The figure shows three views and two pictorial views of one solid part (mm, origin at its lowest corner). Answer the questions. A direction names the side the tool comes from. Coordinates: 2 decimals unless noted, no trailing zeros. Write each loop counter-clockwise with the first axis right and the second up, starting at its lowest first coordinate (ties: lowest second). Pieces come first, ordered by that corner, then holes.
Item 1: Section C-C (x = 63.5) is taken. Give the vertices of the cut face in (y, z), then the cut area to 3 significant figures.
Item 2: Section B-B (z = 24) is taken. Give the vertices of the cut face in (x, y), then the cut area to 3 significant figures.
Item 3: Each of these flat-tipped pins is pushed along its axis until it touches: P1, Ø16.5, axis at x = 12.7, y = 12.7, coming from the +Z side; P2, Ø2, axis at x = 53, z = 43.5, coming from the +Y side; P3, Ø10, axis at y = 47.5, z = 36.5, coming from the +X side. Where does it stop, or does it pass through?
Item 4: Determine the mould class of the marked faces 1, 2, 3 and 4 for opening direction Y: released by +Y, released by -Y, zero draft, split by the parting line, or undercut.
Item 5: A tool of negligible diameter and unlimited length cuts with its end or side. For the marked faces 5 and 6, from which of +Z, -Z, +X, -X, +Y, -Y can it reach the whole face along a straight path? Write none if from no direction.
Item 6: Section A-A (x = 114.3) is taken. Give the vertices of the cut face in (y, z).
Item 7: Section D-D (z = 44.5) is taken. Give the vertices of the cut face in (x, y), then the cut area to 3 significant figures.
Item 8: Straight lines are drawn through the part: probe 1 along Y at (x, z) = (114.3, 6.75); probe 2 along X at (y, z) = (63, 17); probe 3 along Z at (x, y) = (78, 49). For each, find the intervals that lie inside material, in ascending order.
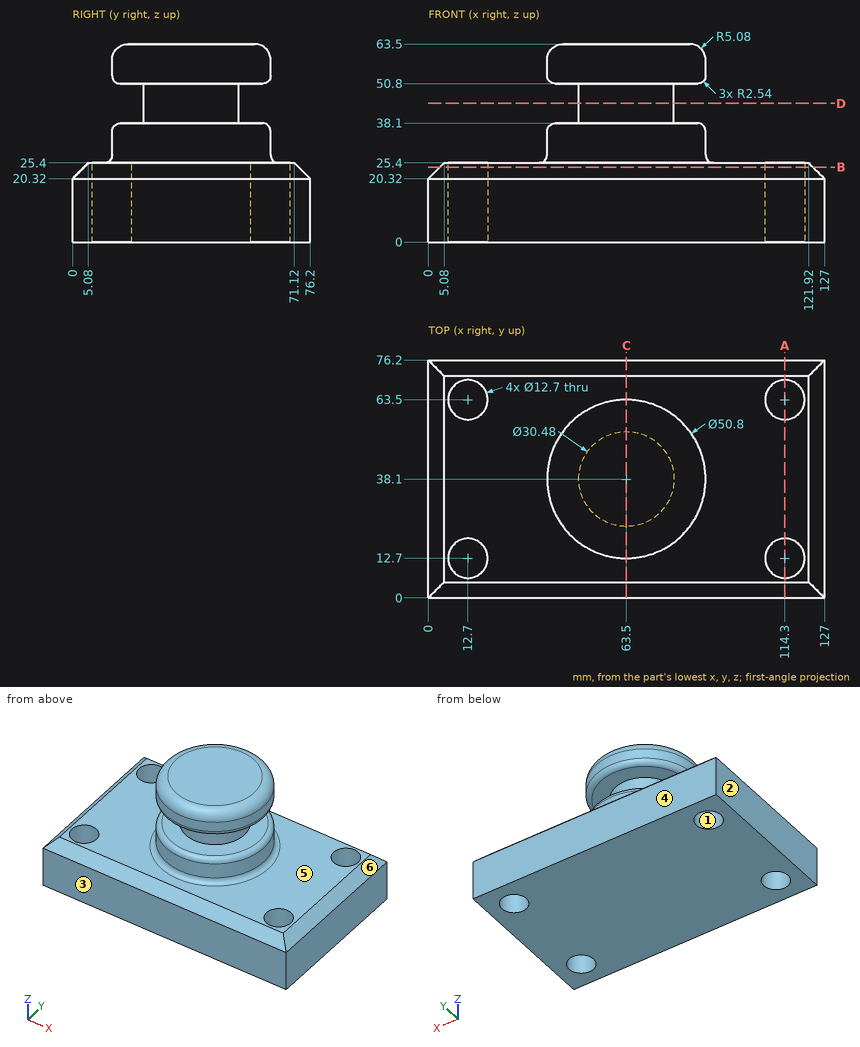
Established:
1. outline: (0, 0) - (76.2, 0) - (76.2, 20.32) - (71.12, 25.4) - (66.04, 25.4) arc R2.54 cw to (63.5, 27.94) - (63.5, 35.56) arc R2.54 ccw to (60.96, 38.1) - (53.34, 38.1) - (53.34, 50.8) - (60.96, 50.8) arc R2.54 ccw to (63.5, 53.34) - (63.5, 58.42) arc R5.08 ccw to (58.42, 63.5) - (17.78, 63.5) arc R5.08 ccw to (12.7, 58.42) - (12.7, 53.34) arc R2.54 ccw to (15.24, 50.8) - (22.86, 50.8) - (22.86, 38.1) - (15.24, 38.1) arc R2.54 ccw to (12.7, 35.56) - (12.7, 27.94) arc R2.54 cw to (10.16, 25.4) - (5.08, 25.4) - (0, 20.32) - close
1. area: 3,570 mm2
2. outline: (3.68, 3.68) - (123.32, 3.68) - (123.32, 72.52) - (3.68, 72.52) - close; hole circle Ø12.7 at (12.7, 12.7); hole circle Ø12.7 at (12.7, 63.5); hole circle Ø12.7 at (114.3, 12.7); hole circle Ø12.7 at (114.3, 63.5)
2. area: 7,730 mm2
3. P1: stops at z = 25.4
3. P2: stops at y = 50.02
3. P3: stops at x = 88.5
4. face 1: undercut
4. face 2: zero draft
4. face 3: released by -Y
4. face 4: released by +Y
5. face 5: +Z
5. face 6: +Z, +X, +Y, -Y
6. outline: (0, 0) - (6.35, 0) - (6.35, 25.4) - (5.08, 25.4) - (0, 20.32) - close; (19.05, 0) - (57.15, 0) - (57.15, 25.4) - (19.05, 25.4) - close; (69.85, 0) - (76.2, 0) - (76.2, 20.32) - (71.12, 25.4) - (69.85, 25.4) - close
7. outline: circle Ø30.48 at (63.5, 38.1)
7. area: 730 mm2
8. probe 1: y = 0 to 6.35, 19.05 to 57.15, 69.85 to 76.2
8. probe 2: x = 0 to 6.37, 19.03 to 107.97, 120.63 to 127
8. probe 3: z = 0 to 38.1, 50.8 to 63.5
